```python
from build123d import *

# Parameters (mm, degrees)
BOSS_EXTRUDE5_START      = -4.7625
BOSS_EXTRUDE5_DEPTH      = 9.525
SKETCH6_R                = 1.778
CUT_EXTRUDE3_DEPTH       = 504.713812734
SKETCH10_R               = 1.778
CUT_EXTRUDE6_DEPTH       = 502.305899638
CUT_EXTRUDE11_DEPTH      = 3.556
CUT_EXTRUDE11_DEPTH_BACK = 499.029405252
SKETCH12_R               = 3.175
SKETCH13_R               = 1.778
CUT_EXTRUDE12_DEPTH      = 500.236768439
SKETCH14_R               = 3.175
CUT_EXTRUDE13_DEPTH      = 19.05
CUT_EXTRUDE14_DEPTH      = 3.556
CUT_EXTRUDE14_DEPTH_BACK = 502.047726259
SKETCH16_R               = 3.175
CUT_EXTRUDE15_START      = -9.525
CUT_EXTRUDE15_DEPTH      = 9.525


# Read off the part's stored shape, not the designer's step: Boss-Extrude5, Cut-Extrude15
with BuildPart() as part:
    # Boss-Extrude5 outline → Boss-Extrude5 (new body)
    with BuildSketch(Plane(origin=(0, 0, 4.097149242), x_dir=(-1, 0, 0), z_dir=(0, 0, -1)).offset(BOSS_EXTRUDE5_START)):
        with BuildLine():
            Line((275.968535621, -57.45686485), (268.466452075, -56.806773151))
            Line((268.466452075, -56.806773151), (268.19701998, -59.916030026))
            add(Edge.make_bspline(
                [(268.19701998, -59.916030026), (268.301513894, -59.925084927), (271.460895726, -60.19858153), (277.676804899, -60.720078346), (287.936274788, -61.527892452), (307.662146031, -62.961314107), (336.878063452, -64.674562273), (362.299459592, -65.630758689), (375.34563844, -65.980821156), (376.009263562, -65.998351659), (376.506986395, -66.011361482), (376.838803336, -66.019942665), (377.004712591, -66.024210248)],
                knots=[0.337983756, 0.337983756, 0.337983756, 0.337983756, 0.338649363, 0.358108739, 0.377568116, 0.403957689, 0.483619427, 0.563281166, 0.565387596, 0.566440812, 0.567494027, 0.568547243, 0.568547243, 0.568547243, 0.568547243], degree=3))
            ThreePointArc((377.004712591, -66.024210248), (434.484295389, -74.49501479), (488.276522854, -96.450725494))
            ThreePointArc((488.276522854, -96.450725494), (494.19519795, -94.762435803), (492.499924864, -88.845757162))
            ThreePointArc((492.499924864, -88.845757162), (472.347982204, -65.669309605), (471.824439099, -34.961421092))
            ThreePointArc((471.824439099, -34.961421092), (471.408544547, -32.082865726), (468.823110549, -30.750731982))
            Line((468.823110549, -30.750731982), (459.298110549, -30.750731982))
            ThreePointArc((459.298110549, -30.750731982), (456.664489609, -32.15241144), (456.356218194, -35.119840174))
            ThreePointArc((456.356218194, -35.119840174), (459.038549003, -44.793404021), (459.444428928, -54.823757832))
            ThreePointArc((459.444428928, -54.823757832), (457.624194748, -58.605108853), (453.717728119, -60.138531982))
            Line((453.717728119, -60.138531982), (423.379813153, -60.138532201))
            add(Edge.make_bspline(
                [(384.561436501, -59.721923859), (385.342635212, -59.738787815), (398.280332925, -60.009594345), (411.224581778, -60.140000907), (423.379813153, -60.138532201)],
                knots=[0.584240942, 0.584240942, 0.584240942, 0.584240942, 0.589217583, 0.666659111, 0.666659111, 0.666659111, 0.666659111], degree=3))
            ThreePointArc((384.561436501, -59.721923859), (381.203597368, -58.363400914), (379.593520206, -55.118663672))
            ThreePointArc((379.593520206, -55.118663672), (380.07016651, -44.713375232), (383.473239108, -34.868766752))
            ThreePointArc((383.473239108, -34.868766752), (383.382771388, -31.793732831), (380.728271975, -30.238853129))
            add(Edge.make_bspline(
                [(371.223837985, -29.983824335), (374.39174563, -30.077394979), (377.559905672, -30.162404856), (380.728271975, -30.238853129)],
                knots=[0.554073124, 0.554073124, 0.554073124, 0.554073124, 0.574595609, 0.574595609, 0.574595609, 0.574595609], degree=3))
            ThreePointArc((371.223837985, -29.983824335), (368.489785186, -31.39412107), (368.234547952, -34.459873245))
            ThreePointArc((368.234547952, -34.459873245), (371.104790651, -44.472811018), (371.022751, -54.88868758))
            ThreePointArc((371.022751, -54.88868758), (369.240986237, -58.042412825), (365.815125645, -59.218910906))
            add(Edge.make_bspline(
                [(302.861547137, -56.088038468), (305.811031553, -56.28688123), (317.379618611, -57.037979008), (337.579863558, -58.152389447), (355.620822681, -58.885705677), (365.034145822, -59.193857367), (365.815125645, -59.218910906)],
                knots=[0.410604965, 0.410604965, 0.410604965, 0.410604965, 0.429432973, 0.484442087, 0.539451201, 0.544427837, 0.544427837, 0.544427837, 0.544427837], degree=3))
            ThreePointArc((302.861547137, -56.088038468), (298.580567699, -54.010676189), (296.944813444, -49.54228442))
            ThreePointArc((296.944813444, -49.54228442), (298.48456489, -40.039989376), (302.371739219, -31.23349624))
            ThreePointArc((302.371739219, -31.23349624), (302.471812822, -28.129850677), (299.876260243, -26.425228339))
            add(Edge.make_bspline(
                [(290.39363306, -25.733255912), (293.55387775, -25.972454095), (296.714768824, -26.203112639), (299.876260243, -26.425228339)],
                knots=[0.379346778, 0.379346778, 0.379346778, 0.379346778, 0.39986924, 0.39986924, 0.39986924, 0.39986924], degree=3))
            ThreePointArc((290.39363306, -25.733255912), (287.546704938, -27.087400093), (287.270368838, -30.227837094))
            ThreePointArc((287.270368838, -30.227837094), (290.158173856, -39.457070008), (290.605029929, -49.117218954))
            ThreePointArc((290.605029929, -49.117218954), (288.384368096, -53.437608207), (283.759752935, -54.924227487))
            Line((283.759752935, -54.924227487), (276.225556942, -54.309054203))
            Line((276.225556942, -54.309054203), (275.968535621, -57.45686485))
        make_face()
    extrude(amount=BOSS_EXTRUDE5_DEPTH)

    # Sketch6 → Cut-Extrude3 (cut, through all)
    with BuildSketch(Plane(origin=(0.329719812, -4.518402653, 0), x_dir=(0.9973480826532571, 0.07277913181587167, 0), z_dir=(-0.07277913181587167, 0.9973480826532571, 0))):
        with Locations(Location((-296.227216633, -4.097149242, 0), (0, 0, 180))):
            Circle(SKETCH6_R)
    extrude(amount=-CUT_EXTRUDE3_DEPTH, mode=Mode.SUBTRACT)

    # Sketch10 → Cut-Extrude6 (cut, through all)
    with BuildSketch(Plane(origin=(0.536880971, -20.008501524, 0), x_dir=(0.9996401989225796, 0.02682298823818541, 0), z_dir=(-0.02682298823818541, 0.9996401989225796, 0))):
        with Locations(Location((-376.648454476, -4.097149242, 0), (0, 0, 180))):
            Circle(SKETCH10_R)
    extrude(amount=-CUT_EXTRUDE6_DEPTH, mode=Mode.SUBTRACT)

    # Sketch12 → Cut-Extrude11 (cut, two sides: drawn at the far end of the back side and taken through both)
    with BuildSketch(Plane(origin=(1.49547556, -55.733443025, 0), x_dir=(0.9996401989225796, 0.02682298823818541, 0), z_dir=(-0.02682298823818541, 0.9996401989225796, 0)).offset(-CUT_EXTRUDE11_DEPTH_BACK)):
        with Locations(Location((-376.656171029, -4.097149242, 0), (0, 0, 180))):
            Circle(SKETCH12_R)
    extrude(amount=CUT_EXTRUDE11_DEPTH + CUT_EXTRUDE11_DEPTH_BACK, mode=Mode.SUBTRACT)

    # Sketch13 → Cut-Extrude12 (cut, through all)
    with BuildSketch(Plane(origin=(0, -30.750731982, 0), x_dir=(1, 0, 0), z_dir=(0, 1, 0))):
        with Locations(Location((-464.060610549, -4.097149242, 0), (0, 0, 270))):
            Circle(SKETCH13_R)
    extrude(amount=-CUT_EXTRUDE12_DEPTH, mode=Mode.SUBTRACT)

    # Sketch14 → Cut-Extrude13 (cut)
    with BuildSketch(Plane(origin=(0, -67.072731982, 0), x_dir=(1, 0, 0), z_dir=(0, 1, 0))):
        with Locations(Location((-464.060610549, -4.097149242, 0), (0, 0, 270))):
            Circle(SKETCH14_R)
    extrude(amount=-CUT_EXTRUDE13_DEPTH, mode=Mode.SUBTRACT)

    # Sketch16 → Cut-Extrude14 (cut, two sides: drawn at the far end of the back side and taken through both)
    with BuildSketch(Plane(origin=(2.825316242, -38.717468408, 0), x_dir=(0.9973480826532571, 0.07277913181587167, 0), z_dir=(-0.07277913181587167, 0.9973480826532571, 0)).offset(-CUT_EXTRUDE14_DEPTH_BACK)):
        with Locations(Location((-296.227216633, -4.097149242, 0), (0, 0, 180))):
            Circle(SKETCH16_R)
    extrude(amount=CUT_EXTRUDE14_DEPTH + CUT_EXTRUDE14_DEPTH_BACK, mode=Mode.SUBTRACT)

    # Cut-Extrude15 outline → Cut-Extrude15 (cut)
    with BuildSketch(Plane.XY.offset(8.859649242).offset(CUT_EXTRUDE15_START)):
        with BuildLine():
            ThreePointArc((-455.130446271, -77.765392477), (-441.88722837, -73.326674178), (-428.412276206, -69.65098313))
            ThreePointArc((-428.412276206, -69.65098313), (-425.977962572, -66.146304208), (-429.169209779, -63.313531984))
            Line((-429.169209779, -63.313531984), (-456.269428929, -63.313531984))
            ThreePointArc((-456.269428929, -63.313531984), (-458.514492959, -64.243467954), (-459.444428928, -66.488531984))
            Line((-459.444428928, -66.488531984), (-459.444428928, -74.753979193))
            ThreePointArc((-459.444428928, -74.753979193), (-458.072640456, -77.384523639), (-455.130446271, -77.765392477))
        make_face()
    extrude(amount=CUT_EXTRUDE15_DEPTH, mode=Mode.SUBTRACT)


solid = part.part
```
Can you work these out from the model? Positions are in its coordinate system, mm. A direction names the side the tool comes from. Coordinates: 2 decimals unless noted, no trailing zeros. Write each loop counter-clockwise with the first axis right and the second up, starting at its lowest first coordinate (ties: lowest second). Pieces come first, ordered by that corner, then holes. Notation, with made-up numbers: (12.5, 47) - (68.5, 47) arc R21 ccw to (68.5, 67) - close; hole circle Ø2 at (-30, 34). An arc over 180 degrees is marked (long way). Return JSON: item names as keys, results as strings.
Q1. If we section it at B-B (y = -38): Count the separate pieces of the cut face and the enclosed holes in it, then the cut area to 3 significant figures.
Computed values:
{"separate pieces": "3", "enclosed holes": "3", "area": "305 mm2"}
Q2. Thinking about a two-plate mould opening in Y: for faces 4 (the flat face through (-443, -63.314, 4)), 5 (the flat face through (-389, -64, 8.86)), 6 (the cylindrical face through (-433.7, -74.28, 4.16)), which applies, +Y half, -Y half, draft (parallel to the pull), parting line (faces both ways), or undercut?
Computed values:
{"face 4": "undercut", "face 5": "draft", "face 6": "-Y half"}
Q3. On a 3-axis mill with a long thin cutter (end or side, diameter ignored), from which of +Z, -Z, +X, -X, +Y, -Y can I reach the whole of each face in a straight line? I mean faces 1 (the cylindrical face through (-298.627, -54.061, 4.164)), 2 (the cylindrical face through (-373.775, -45.926, 4.175)), 3 (the flat face through (-272.27, -57.136, 4.164)). Say none if no direction works.
Computed values:
{"face 1": "+Z, -Z", "face 2": "none", "face 3": "+Z, -Z, +Y"}
Q4. I'm going to push flat-ended pins straight in: pin 1 Ø5 at (x, z) = (-445, 3.5) entering from -Y; pin 2 Ø4 at (x, z) = (-464.06, 4.1) entering from +Y; pin 3 Ø5 at (x, z) = (-429, 1) entering from +Y. Where does each tip first touch, or does it pass through?
Computed values:
{"pin 1": "stops at y = -78.45", "pin 2": "stops at y = -30.75", "pin 3": "stops at y = -60.14"}
Q5. Please list where these lines run through material, in increasing order: L1, parallel to X at y = -47, z = 4; L2, parallel to X at y = -44, z = 4; L3, parallel to X at y = -85, z = 5.5. Write a range as from..to.
Computed values:
{"L1": "x = -469.45..-465.84, -462.29..-459.33, -379.71..-377.3, -373.75..-371.36, -297.11..-295.37, -291.81..-290.72", "L2": "x = -469.72..-465.84, -462.29..-458.91, -380.21..-377.38, -373.83..-371.04, -297.54..-295.58, -292.02..-290.68", "L3": "x = -486.68..-466.91"}
Q6. If we section it at A-A (x = -443): Please give me the cut outline in (y, z), then the cut area to 3 significant figures.
Computed values:
{"outline": "(-76.99, -0.67) - (-73.67, -0.67) - (-73.67, 8.86) - (-76.99, 8.86) - close; (-63.31, -0.67) - (-60.14, -0.67) - (-60.14, 8.86) - (-63.31, 8.86) - close", "area": "61.9 mm2"}
